Build history of the part. All positions in model axes, mm. Face numbers are marked on the shaded views. A direction names the side the tool comes from. Give positions to 0.01 mm unless a question says otherwise; leave off trailing zeros. Write each loop counter-clockwise with the first axis right and the second up, starting at its lowest first coordinate (ties: lowest second). Pieces come first, ordered by that corner, then holes.
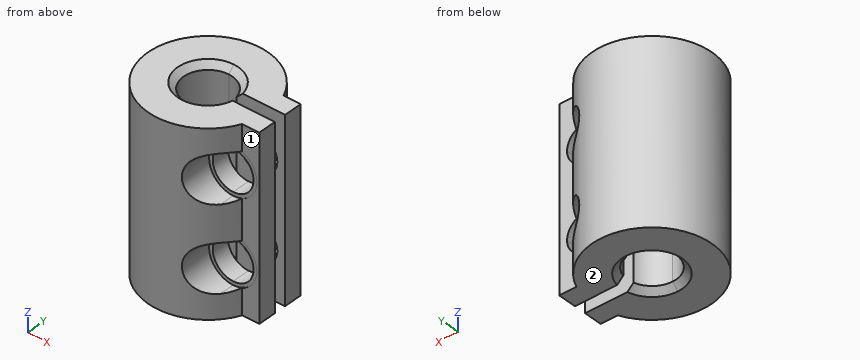
from build123d import *

# Parameters (mm, degrees)
F2_DEPTH = 15
F3_DEPTH = 5
F4_DEPTH = 5
F7_DEPTH = 3
F8_SIZE  = 0.5


with BuildPart() as f2:
    # F0 (on Top) → F2 (new body)
    with BuildSketch(Plane.XY):
        with BuildLine():
            ThreePointArc((0, -2.025), (-2.025, 0), (0, 2.025))
            Line((0, 2.025), (4.5715834237, 2.025))
            ThreePointArc((4.5715834237, 2.025), (-5, 0), (4.5715834237, -2.025))
            Line((4.5715834237, -2.025), (0, -2.025))
        make_face()
        with BuildLine():
            Line((4.5715834237, 2.025), (0, 2.025))
            ThreePointArc((0, 2.025), (1.2426031144, 1.5989254204), (1.9623009453, 0.5))
            Line((1.9623009453, 0.5), (4.9749371855, 0.5))
            ThreePointArc((4.9749371855, 0.5), (4.8337790791, 1.2785068691), (4.5715834237, 2.025))
        make_face()
        with BuildLine():
            ThreePointArc((1.9623009453, -0.5), (1.2426031144, -1.5989254204), (0, -2.025))
            Line((0, -2.025), (4.5715834237, -2.025))
            ThreePointArc((4.5715834237, -2.025), (4.8337790791, -1.2785068691), (4.9749371855, -0.5))
            Line((4.9749371855, -0.5), (1.9623009453, -0.5))
        make_face()
        with BuildLine():
            Line((6, 2.025), (4.5715834237, 2.025))
            ThreePointArc((4.5715834237, 2.025), (4.8337790791, 1.2785068691), (4.9749371855, 0.5))
            Line((4.9749371855, 0.5), (5.5474806577, 0.5))
            Line((5.5474806577, 0.5), (6, 0.5))
            Line((6, 0.5), (6, 2.025))
        make_face()
        with BuildLine():
            ThreePointArc((4.9749371855, -0.5), (4.8337790791, -1.2785068691), (4.5715834237, -2.025))
            Line((4.5715834237, -2.025), (6, -2.025))
            Line((6, -2.025), (6, -0.5))
            Line((6, -0.5), (5.5474806577, -0.5))
            Line((5.5474806577, -0.5), (4.9749371855, -0.5))
        make_face()
    extrude(amount=F2_DEPTH)

    # F1 (on Front) → F3 (cut)
    with BuildSketch(Plane.XZ):
        with BuildLine():
            ThreePointArc((5.35, 11), (2.7039844892, 12.0960155108), (3.8, 9.45))
            ThreePointArc((3.8, 9.45), (4.8960155108, 9.9039844892), (5.35, 11))
        make_face()
        with BuildLine():
            Line((3.8, 4), (3.8, 2.45))
            ThreePointArc((3.8, 2.45), (4.8960155108, 2.9039844892), (5.35, 4))
            ThreePointArc((5.35, 4), (4.8960155108, 5.0960155108), (3.8, 5.55))
            Line((3.8, 5.55), (3.8, 4))
        make_face()
        with BuildLine():
            ThreePointArc((3.8, 5.55), (2.25, 4), (3.8, 2.45))
            Line((3.8, 2.45), (3.8, 4))
            Line((3.8, 4), (3.8, 5.55))
        make_face()
    extrude(amount=-F3_DEPTH, mode=Mode.SUBTRACT)

    # F1 (on Front) → F4 (cut)
    with BuildSketch(Plane.XZ):
        with BuildLine():
            ThreePointArc((5.5, 11), (2.597918472, 12.202081528), (3.8, 9.3))
            ThreePointArc((3.8, 9.3), (5.002081528, 9.797918472), (5.5, 11))
        make_face()
        with BuildLine():
            ThreePointArc((5.35, 11), (4.8960155108, 9.9039844892), (3.8, 9.45))
            ThreePointArc((3.8, 9.45), (2.7039844892, 12.0960155108), (5.35, 11))
        make_face(mode=Mode.SUBTRACT)
        with BuildLine():
            ThreePointArc((5.35, 11), (2.7039844892, 12.0960155108), (3.8, 9.45))
            ThreePointArc((3.8, 9.45), (4.8960155108, 9.9039844892), (5.35, 11))
        make_face()
        with BuildLine():
            Line((3.8, 4), (3.8, 2.45))
            ThreePointArc((3.8, 2.45), (4.8960155108, 2.9039844892), (5.35, 4))
            ThreePointArc((5.35, 4), (4.8960155108, 5.0960155108), (3.8, 5.55))
            Line((3.8, 5.55), (3.8, 4))
        make_face()
        with BuildLine():
            ThreePointArc((3.8, 5.55), (2.25, 4), (3.8, 2.45))
            Line((3.8, 2.45), (3.8, 4))
            Line((3.8, 4), (3.8, 5.55))
        make_face()
        with BuildLine():
            Line((3.8, 2.45), (3.8, 2.3))
            ThreePointArc((3.8, 2.3), (5.002081528, 2.797918472), (5.5, 4))
            ThreePointArc((5.5, 4), (5.002081528, 5.202081528), (3.8, 5.7))
            Line((3.8, 5.7), (3.8, 5.55))
            ThreePointArc((3.8, 5.55), (4.8960155108, 5.0960155108), (5.35, 4))
            ThreePointArc((5.35, 4), (4.8960155108, 2.9039844892), (3.8, 2.45))
        make_face()
        with BuildLine():
            ThreePointArc((3.8, 5.7), (2.1, 4), (3.8, 2.3))
            Line((3.8, 2.3), (3.8, 2.45))
            ThreePointArc((3.8, 2.45), (2.25, 4), (3.8, 5.55))
            Line((3.8, 5.55), (3.8, 5.7))
        make_face()
    extrude(amount=F4_DEPTH, mode=Mode.SUBTRACT)

    # F6 (on offset) → F7 (cut)
    with BuildSketch(Plane.XZ.offset(5)):
        with BuildLine():
            ThreePointArc((5.8, 11), (2.3857864376, 12.4142135624), (3.8, 9))
            ThreePointArc((3.8, 9), (5.2142135624, 9.5857864376), (5.8, 11))
        make_face()
        with BuildLine():
            ThreePointArc((3.8, 6), (1.8, 4), (3.8, 2))
            Line((3.8, 2), (3.8, 4))
            Line((3.8, 4), (3.8, 6))
        make_face()
        with BuildLine():
            Line((3.8, 4), (3.8, 2))
            ThreePointArc((3.8, 2), (5.2142135624, 2.5857864376), (5.8, 4))
            ThreePointArc((5.8, 4), (5.2142135624, 5.4142135624), (3.8, 6))
            Line((3.8, 6), (3.8, 4))
        make_face()
    extrude(amount=-F7_DEPTH, mode=Mode.SUBTRACT)

    # F8
    f8_edges = [f2.edges().sort_by_distance(p)[0] for p in [
        (-2.025, 0, 15),
        (-2.025, 0, 0),
    ]]
    chamfer(f8_edges, length=F8_SIZE)


solid = f2.part
1. Saw through at C-C on z = 7.75. Give the cut face in (x, y) (3 decimals), plus the area to 3 significant figures.
2. Drill centre lines: line 1 along Z through (x, y) = (3.8, 1.5); line 2 along Z through (x, y) = (3.8, -1.5); line 3 along X through (y, z) = (1.7, 11). Where is each one in solid material? Low to high.
3. Saw through at A-A on x = 3.25. Count the separate pieces of the cut face and the enclosed holes in it, plus the area to 3 significant figures.
4. 3-axis set-ups, long thin cutter, end or side, ignore diameter. For the marked faces 1 and 2: which of +Z, -Z, +X, -X, +Y, -Y reach the whole face in a straight line?
5. Saw through at B-B on y = 0. Give the cut face in (x, z) (3 decimals).
6. Saw through at D-D on y = 3.75. Give the cut face in (x, z).
7. Drop flat-ended pins along their axis: pin 1 (1.6 mm diameter, centred on x = 5.5, z = 5.5, fed in from +Y) (3 decimals); pin 2 (2 mm diameter, centred on x = 3.5, z = 6, fed in from +Y); pin 3 (2 mm diameter, centred on x = -2, z = 11, fed in from +Y). Give the stop position or say it passes through.
Outcome:
1. outline: (1.962, -0.5) arc R2.025 cw (long way) to (1.962, 0.5) - (6, 0.5) - (6, 2.025) - (4.572, 2.025) arc R5 ccw (long way) to (4.572, -2.025) - (6, -2.025) - (6, -0.5) - close
1. area: 66.3 mm2
2. line 1: z = 0 to 2.45, 5.55 to 9.45, 12.55 to 15
2. line 2: z = 0 to 2.3, 5.7 to 9.3, 12.7 to 15
2. line 3: x = -4.7 to -1.1, 1.1 to 2.25, 5.35 to 6
3. separate pieces: 6
3. enclosed holes: 0
3. area: 56.4 mm2
4. face 1: +Z, -Z, +X, -Y
4. face 2: -Z, +X, -X, +Y, -Y
5. outline: (-5, 0) - (-2.525, 0) - (-2.025, 0.5) - (-2.025, 14.5) - (-2.525, 15) - (-5, 15) - close
6. outline: (-3.31, 0) - (3.31, 0) - (3.31, 2.53) arc R1.55 cw to (3.31, 5.47) - (3.31, 9.53) arc R1.55 cw to (3.31, 12.47) - (3.31, 15) - (-3.31, 15) - close
7. pin 1: stops at y = 2.025
7. pin 2: stops at y = 4.33
7. pin 3: stops at y = 4.9
